from build123d import *

# Parameters (mm, degrees)
EXTRUDE_1_DEPTH      = 35
EXTRUDE_1_DEPTH_BACK = 35
SKETCH_1_R           = 25
SKETCH_2_W           = 50
SKETCH_2_H           = 50
EXTRUDE_2_DEPTH      = 300
EXTRUDE_3_DEPTH      = 35
EXTRUDE_3_DEPTH_BACK = 35
SKETCH_3_R           = 25


with BuildPart() as part:
    # 草图1 → 凸台-拉伸1 (new, two sides: drawn at the far end of the back side and taken through both)
    with BuildSketch(Plane.XY.offset(-EXTRUDE_1_DEPTH_BACK)):
        Circle(SKETCH_1_R)
    extrude(amount=EXTRUDE_1_DEPTH + EXTRUDE_1_DEPTH_BACK)

    # 草图2 → 凸台-拉伸2 (add)
    with BuildSketch(Plane(origin=(0, 0, 0), x_dir=(1, 0, 0), z_dir=(0, 1, 0))):
        Rectangle(SKETCH_2_W, SKETCH_2_H)
    extrude(amount=EXTRUDE_2_DEPTH)

    # 草图3 → 凸台-拉伸3 (add, two sides: drawn at the far end of the back side and taken through both)
    with BuildSketch(Plane.XY.offset(-EXTRUDE_3_DEPTH_BACK)):
        with Locations((0, 300)):
            Circle(SKETCH_3_R)
    extrude(amount=EXTRUDE_3_DEPTH + EXTRUDE_3_DEPTH_BACK)


solid = part.part
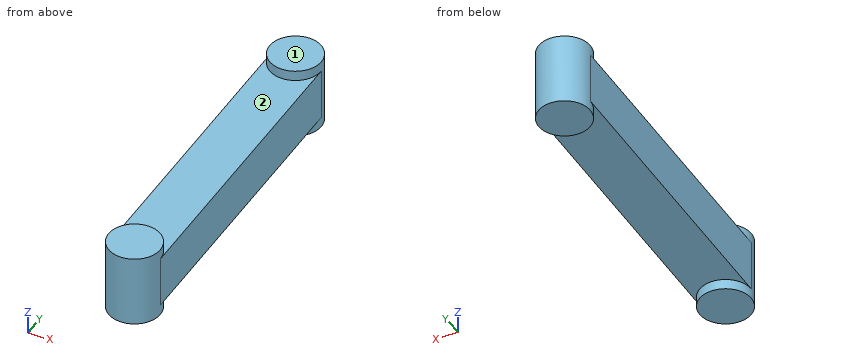
The model under review builds one solid part; all positions refer to its coordinate system, in mm. Face numbers are marked on the shaded views. Coordinates: 2 decimals unless noted, no trailing zeros. Write each loop counter-clockwise with the first axis right and the second up, starting at its lowest first coordinate (ties: lowest second). Pieces come first, ordered by that corner, then holes. Notation, with made-up numbers: (1.5, 5) - (17.5, 5) arc R19 ccw to (17.5, 39) - close; hole circle Ø2 at (-5, 9.25). An arc over 180 degrees is marked (long way). Answer as a JSON object with one key per item and string values. Group by question number.
1. Add section B-B (y = 203). Give the boundary of the cut face in (x, z), plus the area to 3 significant figures.
2. Clearance check with flat-ended pins moving along their axes: pin 1 Ø1.5 at (x, y) = (-15, 245.5) entering from +Z; pin 2 Ø5 at (x, z) = (4, -22.5) entering from +Y; pin 3 Ø1 at (x, z) = (3.5, 23) entering from -Y. State where each tip first meets the part, or that it passes through.
3. Add section C-C (x = 0). Give the boundary of the cut face in (y, z).
4. To check wall thickness, follow probe 1 along Z at (x, y) = (-17.5, 255); probe 2 along Y at (x, z) = (-22.5, -26); probe 3 along Y at (x, z) = (-1.5, -7). State the ranges of each line that lie inside material, in increasing order.
5. Add section D-D (z = 3.5). Give the boundary of the cut face in (x, y).
6. Mouldability with a two-part tool opening along Y and no side actions: class the marked faces 1 and 2 as pulls with the +Y half, pulls with the -Y half, needs draft (parallel to the pull), parting line crosses it, or undercut.
7. Add section A-A (x = -20). Give the boundary of the cut face in (y, z).
Findings:
{
 "1": {"outline": "(-25, -25) - (25, -25) - (25, 25) - (-25, 25) - close", "area": "2,500 mm²"},
 "2": {"pin 1": "z = 25", "pin 2": "y = 324.95", "pin 3": "y = -24.82"},
 "3": {"outline": "(-25, -35) - (25, -35) - (25, -25) - (275, -25) - (275, -35) - (325, -35) - (325, 35) - (275, 35) - (275, 25) - (25, 25) - (25, 35) - (-25, 35) - close"},
 "4": {"probe 1": "-25 to 25", "probe 2": "-10.9 to 10.9, 289.1 to 310.9", "probe 3": "-24.95 to 324.95"},
 "5": {"outline": "(-25, 0) arc R25 ccw to (25, 0) - (25, 300) arc R25 ccw to (-25, 300) - close"},
 "6": {"face 1": "needs draft", "face 2": "undercut"},
 "7": {"outline": "(-15, -35) - (15, -35) - (15, -25) - (285, -25) - (285, -35) - (315, -35) - (315, 35) - (285, 35) - (285, 25) - (15, 25) - (15, 35) - (-15, 35) - close"}
}
